The drawing under review shows one solid part. Ordinate dimensions are in mm from its lowest x, y, z. A direction names the side the tool comes from. Coordinates: 2 decimals unless noted, no trailing zeros. Write each loop counter-clockwise with the first axis right and the second up, starting at its lowest first coordinate (ties: lowest second). Pieces come first, ordered by that corner, then holes. Notation, with made-up numbers: (83, 84.5) -> (132, 84.5) arc R30 cw to (132, 115.5) -> close; hole circle Ø8 at (43, 76). An arc over 180 degrees is marked (long way). One line per question, with ' | ' between items. Start each with the question number.
Q1. Add section C-C on y = 2.6. State the section outline as (x, z) points.
Q2. For the marked faces 5 and 6, list the 3-axis set-ups (+Z, -Z, +X, -X, +Y, -Y) from which the entire face can be reached by the end or side of a thin tool; tool diameter is ignored.
Q3. Wall thickness on probe 1 along X at (y, z) = (1.75, 14); probe 2 along Z at (x, y) = (9, 1.35); probe 3 along Z at (x, y) = (3, 1.8) (1 decimal): over which ranges is each line inside the solid? List them lowest first.
Q4. Draft analysis for pull direction Z (two halves, no side actions). For the marked faces 1, 2, 3 and 4, state which applies: pulls with the +Z half, pulls with the -Z half, needs draft (parallel to the pull), parting line crosses it, or undercut.
Q5. For P1, Ø2, axis at x = 14, z = 7, coming from the +Y side; P2, Ø1.5, axis at x = 11, y = 1.5, coming from the -Z side, all flat-tipped, find the tip position at first contact; note any pin that passes through.
Q6. Add section A-A on z = 10.5. State the section outline as (x, y) points.
Q7. Add section B-B on x = 10. State the section outline as (y, z) points.
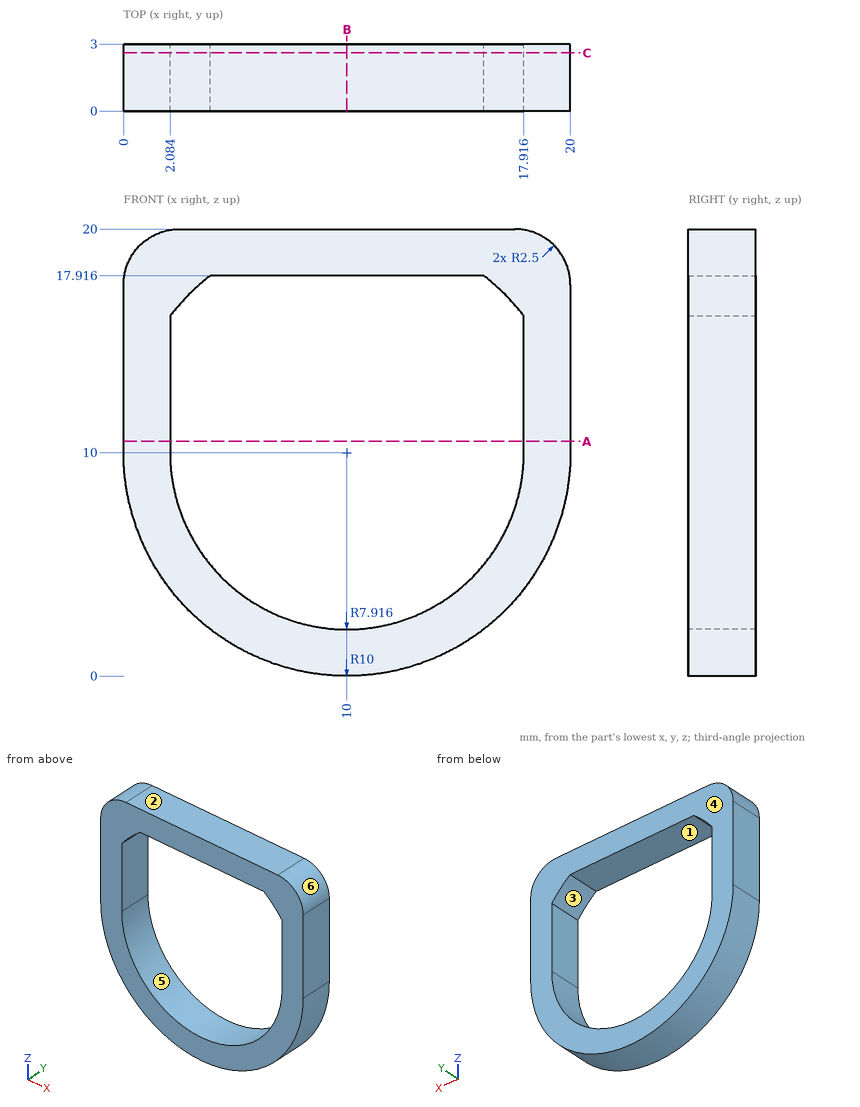
Output values:
1) outline: (0, 10) arc R10 ccw to (20, 10) -> (20, 17.5) arc R2.5 ccw to (17.5, 20) -> (2.5, 20) arc R2.5 ccw to (0, 17.5) -> close; hole (2.08, 10) arc R7.92 ccw to (17.92, 10) -> (17.92, 16.11) arc R10 ccw to (16.11, 17.92) -> (3.89, 17.92) arc R10 ccw to (2.08, 16.11) -> close
2) face 5: +Y, -Y | face 6: +Z, +X, +Y, -Y
3) probe 1: x = 0 to 2.08, 17.92 to 20 | probe 2: z = 0.05 to 2.15, 17.92 to 20 | probe 3: z = 2.9 to 6.3, 17.1 to 20
4) face 1: undercut | face 2: pulls with the +Z half | face 3: undercut | face 4: needs draft
5) P1: passes through | P2: stops at z = 0
6) outline: (0, 0) -> (2.08, 0) -> (2.08, 3) -> (0, 3) -> close; (17.92, 0) -> (20, 0) -> (20, 3) -> (17.92, 3) -> close
7) outline: (0, 0) -> (3, 0) -> (3, 2.08) -> (0, 2.08) -> close; (0, 17.92) -> (3, 17.92) -> (3, 20) -> (0, 20) -> close
